Geometry: see drawing. Coordinates: mm, zero at the bounding-box minimum. A direction names the side the tool comes from. Coordinates: 2 decimals unless noted, no trailing zeros. Write each loop counter-clockwise with the first axis right and the second up, starting at its lowest first coordinate (ties: lowest second). Pieces come first, ordered by that corner, then holes. Notation, with made-up numbers: (52.25, 18) -> (105.25, 18) arc R8 ccw to (105.25, 30) -> close; hole circle Ø4 at (-33.5, -28). An arc over 180 degrees is marked (long way). Answer as a JSON object with one key per item and string values. Group by question number.
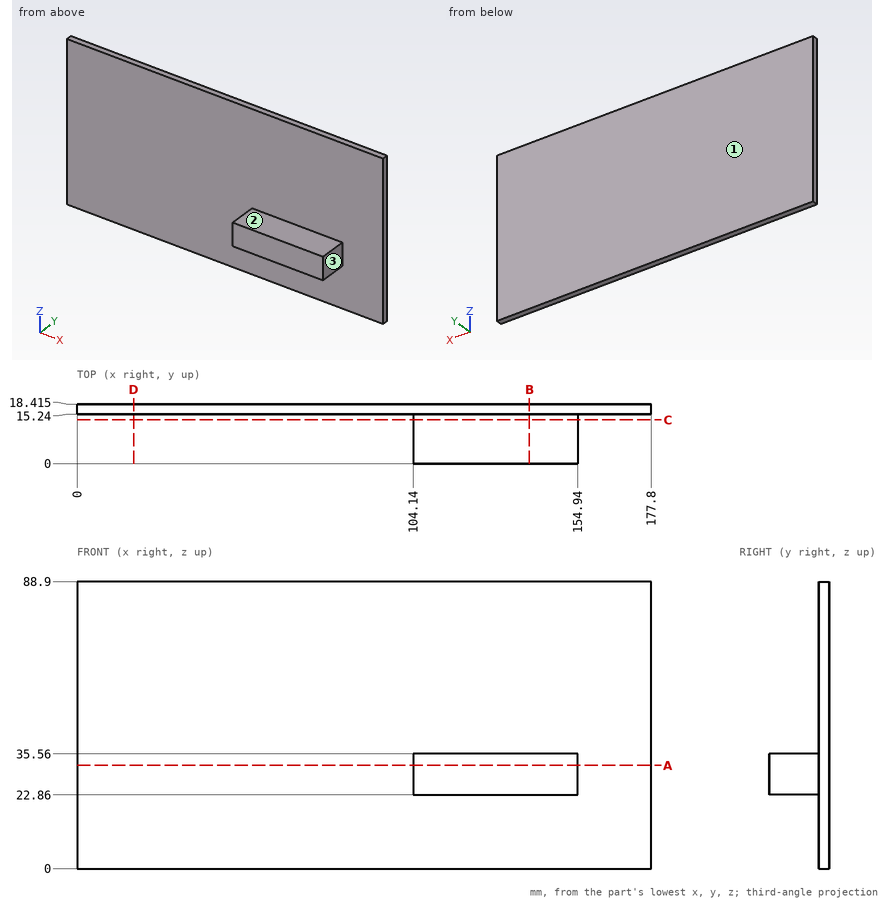
Item 1: Section D-D on x = 17.5. Output: boundary loops of the cut face in (y, z) (3 decimals), then the cut area to 3 significant figures.
Item 2: Contact query for flat-ended pins moving along their axis: pin 1 (4 mm diameter, centred on y = 7, z = 31.5, fed in from -X); pin 2 (8 mm diameter, centred on x = 25, y = 16, fed in from -Z); pin 3 (8 mm diameter, centred on x = 64.5, y = 10, fed in from -Z); pin 4 (6.5 mm diameter, centred on y = 8, z = 29.5, fed in from +X). Output: stop coordinate, or through.
Item 3: Section A-A on z = 32. Output: boundary loops of the cut face in (x, y) (3 decimals), then the cut area to 3 significant figures.
Item 4: Section B-B on x = 140. Output: boundary loops of the cut face in (y, z) (3 decimals).
Item 5: Set-up query: the marked faces 1, 2 and 3. Return all of +Z, -Z, +X, -X, +Y, -Y with unobstructed straight access to the full face (end or side cutting, diameter ignored); none if empty.
Item 6: Ray query, L1, parallel to Y at x = 37, z = 4 (3 decimals); L2, parallel to X at y = 4.5, z = 25; L3, parallel to Z at x = 146, y = 6.25. Return the intervals inside material, ascending. Write a range as [from, to].
Item 7: Section C-C on y = 13.5. Output: boundary loops of the cut face in (x, z).
Answer sheet:
{
 "1": {"outline": "(15.24, 0) -> (18.415, 0) -> (18.415, 88.9) -> (15.24, 88.9) -> close", "area": "282 mm^2"},
 "2": {"pin 1": "stops at x = 104.14", "pin 2": "stops at z = 0", "pin 3": "passes through", "pin 4": "stops at x = 154.94"},
 "3": {"outline": "(0, 15.24) -> (104.14, 15.24) -> (104.14, 0) -> (154.94, 0) -> (154.94, 15.24) -> (177.8, 15.24) -> (177.8, 18.415) -> (0, 18.415) -> close", "area": "1,340 mm^2"},
 "4": {"outline": "(0, 22.86) -> (15.24, 22.86) -> (15.24, 0) -> (18.415, 0) -> (18.415, 88.9) -> (15.24, 88.9) -> (15.24, 35.56) -> (0, 35.56) -> close"},
 "5": {"face 1": "+Z, -Z, +X, -X, +Y", "face 2": "+Z, +X, -X, -Y", "face 3": "+Z, -Z, +X, -Y"},
 "6": {"L1": "y = [15.24, 18.415]", "L2": "x = [104.14, 154.94]", "L3": "z = [22.86, 35.56]"},
 "7": {"outline": "(104.14, 22.86) -> (154.94, 22.86) -> (154.94, 35.56) -> (104.14, 35.56) -> close"}
}
